For this review, take the finished solid that the model builds, in its own axes (mm). A direction names the side the tool comes from. Round coordinates to 2 decimals unless told otherwise and drop trailing zeros. Order: outer loops, then holes, each group sorted by start corner. A loop starts at its lowest first (then second) coordinate and runs counter-clockwise, first axis right, second up. Notation, with made-up numbers: (84.5, 46.25) -> (140.5, 46.25) arc R15 ccw to (140.5, 50.25) -> close; hole circle Ø5 at (14.25, -7). An arc over 180 degrees is marked (long way). Answer in a Markdown table with one row per item.
```python
from build123d import *

# Parameters (mm, degrees)
ESBO_O1_R                = 4.5
RESSALTO_EXTRUS_O1_DEPTH = 50
ESBO_O2_W                = 5
ESBO_O2_H                = 9
RESSALTO_EXTRUS_O2_DEPTH = 6
FILETE1_R                = 2
ESBO_O3_R                = 2.125
CORTE_EXTRUS_O1_DEPTH    = 6


with BuildPart() as part:
    # Esboço1 → Ressalto-extrusão1 (new body)
    with BuildSketch(Plane.XY):
        Circle(ESBO_O1_R)
    extrude(amount=RESSALTO_EXTRUS_O1_DEPTH)

    # Esboço2 → Ressalto-extrusão2 (add)
    with BuildSketch(Plane.XY.offset(50)):
        Rectangle(ESBO_O2_W, ESBO_O2_H)
    extrude(amount=RESSALTO_EXTRUS_O2_DEPTH)

    # Filete1
    # the kernel refuses this fillet: 2 mm, written as the material it takes off along each edge
    with BuildSketch(Plane(origin=(2.5, -4.5, 50), x_dir=(0, 1, 0), z_dir=(0, 0, 1)), Plane(origin=(-2.5, 4.5, 50), x_dir=(0, -1, 0), z_dir=(0, 0, 1)), Plane(origin=(-2.5, -4.5, 50), x_dir=(1, 0, 0), z_dir=(0, 0, 1))) as filete1_piece_1:
        with BuildLine():
            CenterArc((FILETE1_R, FILETE1_R), FILETE1_R, 180, 90)
            Line((0, FILETE1_R), (0, 0))
            Line((0, 0), (FILETE1_R, 0))
        make_face()
    extrude(amount=11, mode=Mode.SUBTRACT)
    with BuildSketch(Plane(origin=(2.5, 4.5, 50), x_dir=(0, -1, 0), z_dir=(0, 0, 1))) as filete1_piece_2:
        with BuildLine():
            CenterArc((FILETE1_R, -FILETE1_R), FILETE1_R, 90, 90)
            Line((0, -FILETE1_R), (0, 0))
            Line((0, 0), (FILETE1_R, 0))
        make_face()
    extrude(amount=11, mode=Mode.SUBTRACT)

    # Esboço3 → Corte-extrusão1 (cut)
    with BuildSketch(Plane.ZY.offset(2.5)):
        with Locations(Location((53, 0, 0), (0, 0, 270))):
            Circle(ESBO_O3_R)
    extrude(amount=-CORTE_EXTRUS_O1_DEPTH, mode=Mode.SUBTRACT)


solid = part.part
```
Q1. Take a section at A-A, the plane y = 0. Write out the cut boundary in (x, z) (3 decimals), then the cut area to 3 significant figures.
Answer key:
| item | result |
|---|---|
| outline | (-4.5, 0) -> (4.5, 0) -> (4.5, 50) -> (2.5, 50) -> (2.5, 50.875) -> (-2.5, 50.875) -> (-2.5, 50) -> (-4.5, 50) -> close; (-2.5, 55.125) -> (2.5, 55.125) -> (2.5, 56) -> (-2.5, 56) -> close |
| area | 459 mm^2 |
Q2. Clearance check with flat-ended pins moving along their axes: pin 1 Ø1 at (x, z) = (-3.5, 15) entering from -Y; pin 2 Ø4 at (y, z) = (0, 54.5) entering from -X; pin 3 Ø2 at (y, z) = (-2.5, 14.5) entering from +X; pin 4 Ø2.5 at (y, z) = (0, 53) entering from +X. State where each tip first meets the part, or that it passes through.
Answer key:
| item | result |
|---|---|
| pin 1 | stops at y = -3.35 |
| pin 2 | stops at x = -2.5 |
| pin 3 | stops at x = 4.24 |
| pin 4 | passes through |
Q3. Take a section at C-C, the plane z = 30.5. Write out the cut boundary in (x, y).
Answer key:
| item | result |
|---|---|
| outline | circle Ø9 at (0, 0) |
Q4. To check wall thickness, follow probe 1 along Z at (x, y) = (-0.7, 0) (3 decimals); probe 2 along Z at (x, y) = (3, -2.5); probe 3 along Y at (x, z) = (0.25, 9.5). State the ranges of each line that lie inside material, in increasing order.
Answer key:
| item | result |
|---|---|
| probe 1 | z = 0 to 50.875, 55.125 to 56 |
| probe 2 | z = 0 to 50 |
| probe 3 | y = -4.49 to 4.49 |
Q5. Take a section at D-D, the plane x = -3.75. Write out the cut boundary in (y, z).
Answer key:
| item | result |
|---|---|
| outline | (-2.49, 0) -> (2.49, 0) -> (2.49, 50) -> (-2.49, 50) -> close |
Q6. Take a section at B-B, the plane y = -3.5. Write out the cut boundary in (x, z), then the cut area to 3 significant figures.
Answer key:
| item | result |
|---|---|
| outline | (-2.83, 0) -> (2.83, 0) -> (2.83, 50) -> (2.23, 50) -> (2.23, 56) -> (-2.23, 56) -> (-2.23, 50) -> (-2.83, 50) -> close |
| area | 310 mm^2 |
Q7. Tool access review of faces 1 (the face through (1.93, 3.9, 52.96)), 2 (the face through (-0.59, 4.46, 24.65)), 3 (the face through (1.9, -3.93, 52.96)): name each direction out of +Z, -Z, +X, -X, +Y, -Y from which nothing blocks a thin tool from reaching the whole face with its end or side.
Answer key:
| item | result |
|---|---|
| face 1 | +Z, +X, +Y |
| face 2 | -Z |
| face 3 | +Z, +X, -Y |
Q8. The part is to be moulded in two halves that separate along Y. For faces 4 (the face through (-2.5, -2.3, 53)), 5 (the face through (-1.93, -3.9, 52.96)), 6 (the face through (-0.035, -0.981, 51.115)), say which applies: +Y half, -Y half, draft (parallel to the pull), parting line (faces both ways), or undercut.
Answer key:
| item | result |
|---|---|
| face 4 | draft |
| face 5 | -Y half |
| face 6 | undercut |
